from build123d import *

# Parameters (mm, degrees)
SKETCH246_R     = 1.85
PAD021_DEPTH    = 5
PAD022_DEPTH    = 3
POCKET017_DEPTH = 5


with BuildPart() as part:
    # Sketch246 → Pad021 (new body)
    with BuildSketch(Plane.XY):
        with BuildLine():
            ThreePointArc((0, 5), (-5, 0), (0, -5))
            Line((0, -5), (24, -5))
            Line((24, -5), (24, 5))
            Line((0, 5), (24, 5))
        make_face()
        Circle(SKETCH246_R, mode=Mode.SUBTRACT)
    extrude(amount=PAD021_DEPTH)

    # Sketch247 (on Face3 of Pad021) → Pad022 (join)
    with BuildSketch(Plane.YZ.offset(24)):
        Polygon((-7, 0), (5, 0), (5, 5), (-5, 11), (-160, 11), (-160, -45), (-7, -45), align=None)
    extrude(amount=PAD022_DEPTH)

    # Sketch248 (on Face11 of Pad022) → Pocket017 (cut)
    with BuildSketch(Plane.YZ.offset(27)):
        with BuildLine():
            ThreePointArc((-144, 7), (-146, 9), (-148, 7))
            Line((-148, 7), (-148, -3))
            ThreePointArc((-148, -3), (-146, -5), (-144, -3))
            Line((-144, 7), (-144, -3))
        make_face()
    extrude(amount=-POCKET017_DEPTH, mode=Mode.SUBTRACT)


with BuildPart() as part_1:
    # Body011 placement: moved
    add(part.part.moved(Location((-96, 98, 234))))


solid = part_1.part
Build history of the part. All positions in model axes, mm. A direction names the side the tool comes from. Round coordinates to 2 decimals unless told otherwise and drop trailing zeros. Loops run counter-clockwise (first coordinate to the right, second up) from the corner with the lowest first, then second, coordinate; pieces in that order, holes last. Notation, with made-up numbers: (-37, -17.75) -> (15, -17.75) arc R22 cw to (15, 6.25) -> close; hole circle Ø6 at (-9, -40). An arc over 180 degrees is marked (long way). One line per item, written item: value. Start each with the question number.
Q1. 3-axis set-ups, long thin cutter, end or side, ignore diameter. For faces 4 (the face through (-84, 93, 236)), 5 (the face through (-87, 98, 239)), 6 (the face through (-70, -50, 236)), 7 (the face through (-71, 91, 211)): which of +Z, -Z, +X, -X, +Y, -Y reach the whole face in a straight line?
Q2. Drop flat-ended pins along their axis: pin 1 Ø1 at (y, z) = (-28.5, 213) entering from -X; pin 2 Ø5 at (x, y) = (-83, 96.5) entering from +Z; pin 3 Ø9.5 at (x, y) = (-79.5, 97) entering from -Z. Give the stop position or say it passes through.
Q3. Cut at B-B on y = 98. List the corners of the cut face in (x, z), plus the area to 4 significant figures.
Q4. Cut at C-C on y = -48. List the corners of the cut face in (x, z).
Q5. Cut at A-A on z = 237. List the corners of the cut face in (x, y), plus the area to 3 significant figures.
Q6. Probe line 1 along Y through (x, z) = (-96, 237); line 2 along X through (y, z) = (98, 235.8); line 3 along X through (y, z) = (-6.5, 222). List the from-to ranges inside material, lowest first.
Q7. Cut at D-D on z = 226. List the corners of the cut face in (x, y), plus the area to 3 significant figures.
Q8. Two-plate mould, pull along Y, no slides. Class faces 1 (the face through (-101, 98, 236)), 2 (the face through (-70, -48, 229)), 3 (the face through (-85, 98, 234)): released by +Y, released by -Y, zero draft, split by the parting line, or undercut.
Computed:
1. face 4: +Z, -Z, -X, -Y
1. face 5: +Z, -X, +Y, -Y
1. face 6: +X, -X
1. face 7: -Z, +X, -X, +Y
2. pin 1: x = -72
2. pin 2: z = 239
2. pin 3: z = 234
3. outline: (-101, 234) -> (-97.85, 234) -> (-97.85, 239) -> (-101, 239) -> close; (-94.15, 234) -> (-69, 234) -> (-69, 242) -> (-72, 242) -> (-72, 239) -> (-94.15, 239) -> close
3. area: 150.5 mm²
4. outline: (-72, 189) -> (-69, 189) -> (-69, 229) -> (-72, 229) -> close; (-72, 243) -> (-69, 243) -> (-69, 245) -> (-72, 245) -> close
5. outline: (-96, 93) -> (-72, 93) -> (-72, -46) -> (-69, -46) -> (-69, 103) -> (-96, 103) arc R5 ccw to start; (-72, -62) -> (-69, -62) -> (-69, -50) -> (-72, -50) -> close; hole circle Ø3.7 at (-96, 98)
5. area: 752 mm²
6. line 1: 93 to 96.15, 99.85 to 103
6. line 2: -101 to -97.85, -94.15 to -69
6. line 3: -72 to -69
7. outline: (-72, -62) -> (-69, -62) -> (-69, 91) -> (-72, 91) -> close
7. area: 459 mm²
8. face 1: split by the parting line
8. face 2: undercut
8. face 3: zero draft
